Autodesk Inventor part; units mm, degrees
ref_plane "YZ Plane" through (0, 0, 0) normal (1, 0, 0) x (0, 1, 0)
ref_plane "XZ Plane" through (0, 0, 0) normal (0, 1, 0) x (-1, 0, 0)
ref_plane "XY Plane" through (0, 0, 0) normal (0, 0, 1) x (1, 0, 0)
sketch "Sketch1" plane through (0, 0, 0) normal (0, 1, 0) x (-1, 0, 0)
  line L0 (-8, 8) -> (-8, -8)
  line L1 (-8, -8) -> (8, -8)
  line L2 (8, -8) -> (8, 8)
  line L3 (8, 8) -> (-8, 8)
  line L4 (-8, 8) -> (8, -8) construction
  line L5 (-8, -8) -> (8, 8) construction
  circle A0 centre (0, 0) radius 4
  dimension "d0" = 16
  dimension "d1" = 8
extrude "Extrusion1" add sketch "Sketch1" along normal mid plane 10
chamfer "Chamfer1" distance 2 angle 45 4 edges at (8, 0, 8) (8, 0, -8) (-8, 0, 8) (-8, 0, -8)
chamfer "Chamfer2" distance 0.5 angle 45 16 edges at (-8, -5, 0) (-7, -5, -7) (0, -5, -8) (8, -5, 0) (7, -5, 7) (0, -5, 8) (-7, -5, 7) (7, -5, -7) (-7, 5, 7) (0, 5, 8) (-8, 5, 0) (-7, 5, -7) (0, 5, -8) (7, 5, -7) (8, 5, 0) (7, 5, 7)
properties part number "Vong_chan" material "Iron, Gray"
Read the model definition and answer for the solid it produces. Units are mm, in the model's axes. Round coordinates to 2 decimals unless told otherwise and drop trailing zeros. Write each loop counter-clockwise with the first axis right and the second up, starting at its lowest first coordinate (ties: lowest second). Pieces come first, ordered by that corner, then holes.
Q1. Find section D-D on z = -7. Determine the outline of the cut face in (x, y).
Values:
outline: (-7, -4.5) - (-6.29, -5) - (6.29, -5) - (7, -4.5) - (7, 4.5) - (6.29, 5) - (-6.29, 5) - (-7, 4.5) - close
Q2. The mould has two halves that part along X. Classify faces 1 (the face through (0, 0, -8)), 2 (the face through (-6.84, 4.75, 6.81)), 3 (the face through (0.867, -0.07, 3.905)), 4 (the face through (8, 0, 0)): released by +X, released by -X, zero draft, split by the parting line, or undercut.
Values:
face 1: zero draft
face 2: released by -X
face 3: undercut
face 4: released by +X
Q3. Find section C-C on z = 0. Determine the outline of the cut face in (x, y), and give its area (3 significant figures).
Values:
outline: (-8, -4.5) - (-7.5, -5) - (-4, -5) - (-4, 5) - (-7.5, 5) - (-8, 4.5) - close; (4, -5) - (7.5, -5) - (8, -4.5) - (8, 4.5) - (7.5, 5) - (4, 5) - close
area: 79.5 mm2
Q4. Find section B-B on y = 3.5. Determine the outline of the cut face in (x, z), and give its area (3 significant figures).
Values:
outline: (-8, -6) - (-6, -8) - (6, -8) - (8, -6) - (8, 6) - (6, 8) - (-6, 8) - (-8, 6) - close; hole circle Ø8 at (0, 0)
area: 198 mm2
Q5. Find section A-A on x = 0. Determine the outline of the cut face in (y, z).
Values:
outline: (-5, -7.5) - (-4.5, -8) - (4.5, -8) - (5, -7.5) - (5, -4) - (-5, -4) - close; (-5, 4) - (5, 4) - (5, 7.5) - (4.5, 8) - (-4.5, 8) - (-5, 7.5) - close
Q6. Straight lines are drawn through the part: line 1 (Z direction, x = 0, y = 2.5); line 2 (X direction, y = -2, z = 1.5); line 3 (X direction, y = 1.5, z = 3). For each, find the intervals that lie inside material, in ascending order.
Values:
line 1: z = -8 to -4, 4 to 8
line 2: x = -8 to -3.71, 3.71 to 8
line 3: x = -8 to -2.65, 2.65 to 8
